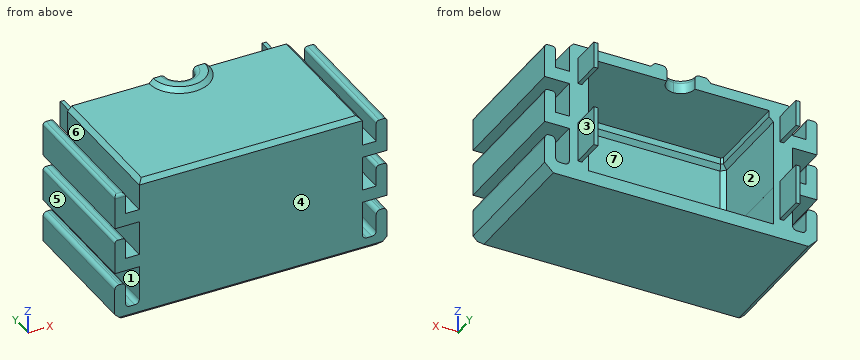
```python
from build123d import *

# Parameters (mm, degrees)
ESQUISSE1_W              = 51.86
ESQUISSE1_H              = 63
BOSS_EXTRU_1_DEPTH       = 20
ENL_V_MAT_EXTRU_1_DEPTH  = 18
ESQUISSE3_W              = 8.7
ESQUISSE3_H              = 3
BOSS_EXTRU_2_DEPTH       = 7
ESQUISSE4_W              = 43
ESQUISSE4_H              = 43
BOSS_EXTRU_3_DEPTH       = 1
CHANFREIN1_SIZE          = 1
ESQUISSE6_R              = 7
BOSS_EXTRU_4_DEPTH       = 5
ENL_V_MAT_EXTRU_2_DEPTH  = 10
BOSS_EXTRU_5_DEPTH       = 63
ESQUISSE9_W              = 2.5
ESQUISSE9_H              = 1
ENL_V_MAT_EXTRU_3_DEPTH  = 63
CHANFREIN3_SIZE          = 1
CONG_1_R                 = 1
CONG_2_R                 = 1
CONG_5_R                 = 0.7
ENL_V_MAT_EXTRU_11_DEPTH = 1.5
ESQUISSE24_W             = 38.565319184
ESQUISSE24_H             = 34.907409987
ENL_V_MAT_EXTRU_16_DEPTH = 74
BOSS_EXTRU_11_REACH      = 71.206
ESQUISSE26_W             = 43.000682915
ESQUISSE26_H             = 8.323167201
ENL_V_MAT_EXTRU_17_DEPTH = 74
ESQUISSE27_W             = 43.00063515
ESQUISSE27_H             = 9
BOSS_EXTRU_12_DEPTH      = 10
BOSS_EXTRU_13_DEPTH      = 1
CHANFREIN4_SIZE          = 1
CHANFREIN5_SIZE          = 1
ESQUISSE29_W             = 0.940494366
ESQUISSE29_H             = 6.11321338
ESQUISSE29_H_2           = 9.278042655
BOSS_EXTRU_14_DEPTH      = 7


with BuildPart() as part:
    # Esquisse1 → Boss.-Extru.1 (new body)
    with BuildSketch(Plane.XY):
        with Locations((25.93, 31.5)):
            Rectangle(ESQUISSE1_W, ESQUISSE1_H)
    extrude(amount=BOSS_EXTRU_1_DEPTH)

    # Esquisse2 → Enlèv. mat.-Extru.1 (cut)
    with BuildSketch(Plane(origin=(0, 0, 0), x_dir=(-1, 0, 0), z_dir=(0, 0, -1))):
        Polygon((-8.231746032, 10), (-43.628253968, 53), (-47.43, 53), (-47.43, 10), align=None)
        Polygon((-4.43, 53), (-43.628253968, 53), (-8.231746032, 10), (-4.43, 10), align=None)
    extrude(amount=-ENL_V_MAT_EXTRU_1_DEPTH, mode=Mode.SUBTRACT)

    # Esquisse3 → Boss.-Extru.2 (add)
    with BuildSketch(Plane(origin=(0, 0, 0), x_dir=(-1, 0, 0), z_dir=(0, 0, -1))):
        with Locations((-8.88, 57.4)):
            Rectangle(ESQUISSE3_W, ESQUISSE3_H)
        with Locations((-42.98, 57.4)):
            Rectangle(ESQUISSE3_W, ESQUISSE3_H)
        with Locations((-42.98, 5.6)):
            Rectangle(ESQUISSE3_W, ESQUISSE3_H)
        with Locations((-8.88, 5.6)):
            Rectangle(ESQUISSE3_W, ESQUISSE3_H)
    extrude(amount=BOSS_EXTRU_2_DEPTH)

    # Esquisse4 → Boss.-Extru.3 (add)
    with BuildSketch(Plane(origin=(0, 0, 18), x_dir=(-1, 0, 0), z_dir=(0, 0, -1))):
        with Locations((-25.93, 31.5)):
            Rectangle(ESQUISSE4_W, ESQUISSE4_H)
    extrude(amount=BOSS_EXTRU_3_DEPTH)

    # Chanfrein1
    chanfrein1_edges = [part.edges().sort_by_distance(p)[0] for p in [
        (47.43, 10, 8.5),
        (47.43, 53, 8.5),
        (4.43, 10, 8.5),
        (4.43, 53, 8.5),
    ]]
    chamfer(chanfrein1_edges, length=CHANFREIN1_SIZE)

    # Esquisse6 → Boss.-Extru.4 (add)
    with BuildSketch(Plane(origin=(0, 0, 17), x_dir=(-1, 0, 0), z_dir=(0, 0, -1))):
        with Locations((-25.93, 31.5)):
            Circle(ESQUISSE6_R)
    extrude(amount=-BOSS_EXTRU_4_DEPTH)

    # Esquisse7 → Enlèv. mat.-Extru.2 (cut)
    with BuildSketch(Plane(origin=(0, 0, 17), x_dir=(-1, 0, 0), z_dir=(0, 0, -1))):
        with BuildLine():
            ThreePointArc((-22.68, 31.5), (-23.631902961, 33.798097039), (-25.93, 34.75))
            Line((-25.93, 34.75), (-25.93, 28.25))
            ThreePointArc((-25.93, 28.25), (-23.631902961, 29.201902961), (-22.68, 31.5))
        make_face()
        with BuildLine():
            Line((-25.93, 28.25), (-25.93, 34.75))
            ThreePointArc((-25.93, 34.75), (-29.18, 31.5), (-25.93, 28.25))
        make_face()
    extrude(amount=-ENL_V_MAT_EXTRU_2_DEPTH, mode=Mode.SUBTRACT)

    # Esquisse8 → Boss.-Extru.5 (add)
    with BuildSketch(Plane(origin=(0, 63, 0), x_dir=(1, 0, 0), z_dir=(0, 1, 0))):
        Polygon((55.06, -3), (55.06, -9), (57.56, -9), (57.56, 0), (51.86, 0), (51.86, -3), align=None)
        Polygon((57.56, -11), (51.86, -11), (51.86, -14), (55.06, -14), (55.06, -20), (57.56, -20), align=None)
        Polygon((0, -3), (0, 0), (-5.7, 0), (-5.7, -9), (-3.2, -9), (-3.2, -3), align=None)
        Polygon((0, -14), (0, -11), (-5.7, -11), (-5.7, -20), (-3.2, -20), (-3.2, -14), align=None)
    extrude(amount=-BOSS_EXTRU_5_DEPTH)

    # Esquisse9 → Enlèv. mat.-Extru.3 (cut)
    with BuildSketch(Plane.XZ):
        with Locations((-4.45, 8.5)):
            Rectangle(ESQUISSE9_W, ESQUISSE9_H)
        with Locations((-4.45, 19.5)):
            Rectangle(ESQUISSE9_W, ESQUISSE9_H)
        with Locations((56.31, 8.5)):
            Rectangle(ESQUISSE9_W, ESQUISSE9_H)
        with Locations((56.31, 19.5)):
            Rectangle(ESQUISSE9_W, ESQUISSE9_H)
    extrude(amount=-ENL_V_MAT_EXTRU_3_DEPTH, mode=Mode.SUBTRACT)

    # Chanfrein3
    chanfrein3_edges = [part.edges().sort_by_distance(p)[0] for p in [
        (46.93, 52.5, 17),
        (4.93, 52.5, 17),
        (46.93, 10.5, 17),
        (4.93, 10.5, 17),
        (25.93, 34.75, 17),
        (4.43, 31.5, 17),
        (25.93, 10, 17),
        (47.43, 31.5, 17),
        (25.93, 53, 17),
    ]]
    chamfer(chanfrein3_edges, length=CHANFREIN3_SIZE)

    # Congé1
    cong_1_edges = [part.edges().sort_by_distance(p)[0] for p in [
        (4.53, 57.4, -7),
        (8.88, 55.9, -7),
        (8.88, 58.9, -7),
        (13.23, 57.4, -7),
        (38.63, 57.4, -7),
        (42.98, 58.9, -7),
        (47.33, 57.4, -7),
        (42.98, 55.9, -7),
        (47.33, 5.6, -7),
        (42.98, 7.1, -7),
        (42.98, 4.1, -7),
        (38.63, 5.6, -7),
        (13.23, 5.6, -7),
        (8.88, 4.1, -7),
        (4.53, 5.6, -7),
        (8.88, 7.1, -7),
    ]]
    fillet(cong_1_edges, radius=CONG_1_R)

    # Congé2
    cong_2_edges = [part.edges().sort_by_distance(p)[0] for p in [
        (25.93, 34.75, 22),
    ]]
    fillet(cong_2_edges, radius=CONG_2_R)

    # Congé5
    cong_5_edges = [part.edges().sort_by_distance(p)[0] for p in [
        (-3.2, 31.5, 19),
        (-5.7, 31.5, 19),
        (-3.2, 31.5, 8),
        (-5.7, 31.5, 8),
        (55.06, 31.5, 8),
        (57.56, 31.5, 8),
        (55.06, 31.5, 19),
        (57.56, 31.5, 19),
        (-4.45, 0, 19),
        (-4.45, 63, 19),
    ]]
    fillet(cong_5_edges, radius=CONG_5_R)

    # Esquisse19 → Enlèv. mat.-Extru.11 (cut)
    with BuildSketch(Plane(origin=(0, 0, 17), x_dir=(-1, 0, 0), z_dir=(0, 0, -1))):
        Polygon((-46.43, 11.414213562), (-46.015786438, 11), (-5.844213562, 11), (-5.43, 11.414213562), (-5.43, 51.585786438), (-5.844213562, 52), (-46.015786438, 52), (-46.43, 51.585786438), align=None)
    extrude(amount=-ENL_V_MAT_EXTRU_11_DEPTH, mode=Mode.SUBTRACT)

    # Esquisse24 → Enlèv. mat.-Extru.16 (cut)
    with BuildSketch(Plane(origin=(57.56, 0, 0), x_dir=(0, 0, -1), z_dir=(1, 0, 0))):
        with Locations((-11.348740569, 48.953704994)):
            Rectangle(ESQUISSE24_W, ESQUISSE24_H)
    extrude(amount=-ENL_V_MAT_EXTRU_16_DEPTH, mode=Mode.SUBTRACT)

    # Boss.-Extru.11: up to this face of the body (flat: up to its plane)
    boss_extru_11_end = Plane(part.part.faces().sort_by_distance((25.97056106, 0, 9.851467598))[0])
    # Esquisse25 → Boss.-Extru.11 (add, up to the picked face)
    with BuildSketch(Plane(origin=(0, 31.5, 0), x_dir=(1, 0, 0), z_dir=(0, 1, 0)), mode=Mode.PRIVATE) as boss_extru_11_sk1:
        with BuildLine():
            Line((47.42936485, 9), (47.43, 0))
            Line((47.43, 0), (51.86, 0))
            Line((51.86, 0), (51.86, 8))
            ThreePointArc((51.86, 8), (52.152893219, 8.707106781), (52.86, 9))
            Line((52.86, 9), (54.06, 9))
            ThreePointArc((54.06, 9), (54.767106781, 8.707106781), (55.06, 8))
            Line((55.06, 8), (55.06, 4))
            ThreePointArc((55.06, 4), (55.352893219, 3.292893219), (56.06, 3))
            Line((56.06, 3), (56.56, 3))
            ThreePointArc((56.56, 3), (57.267106781, 3.292893219), (57.56, 4))
            Line((57.56, 4), (57.56, 10))
            Line((57.56, 10), (55.56, 12))
            Line((55.56, 12), (25.92936485, 12))
            Line((25.92936485, 12), (25.92936485, 9))
            Line((25.92936485, 9), (47.42936485, 9))
        make_face()
    boss_extru_11_tool1 = split(extrude(boss_extru_11_sk1.sketch, amount=-BOSS_EXTRU_11_REACH, mode=Mode.PRIVATE), bisect_by=boss_extru_11_end, keep=Keep.BOTH, mode=Mode.PRIVATE)
    # Esquisse25 → Boss.-Extru.11 (add, up to the picked face)
    with BuildSketch(Plane(origin=(0, 31.5, 0), x_dir=(1, 0, 0), z_dir=(0, 1, 0)), mode=Mode.PRIVATE) as boss_extru_11_sk2:
        with BuildLine():
            Line((4.42936485, 9), (25.92936485, 9))
            Line((25.92936485, 9), (25.92936485, 12))
            Line((25.92936485, 12), (-3.7012703, 12))
            Line((-3.7012703, 12), (-5.7012703, 10))
            Line((-5.7012703, 10), (-5.7012703, 4))
            ThreePointArc((-5.7012703, 4), (-5.408377081, 3.292893219), (-4.7012703, 3))
            Line((-4.7012703, 3), (-4.2012703, 3))
            ThreePointArc((-4.2012703, 3), (-3.494163519, 3.292893219), (-3.2012703, 4))
            Line((-3.2012703, 4), (-3.2012703, 8))
            ThreePointArc((-3.2012703, 8), (-2.908377081, 8.707106781), (-2.2012703, 9))
            Line((-2.2012703, 9), (-1.0012703, 9))
            ThreePointArc((-1.0012703, 9), (-0.294163519, 8.707106781), (-0.0012703, 8))
            Line((-0.0012703, 8), (-0.0012703, 0))
            Line((-0.0012703, 0), (4.4287297, 0))
            Line((4.4287297, 0), (4.42936485, 9))
        make_face()
    boss_extru_11_tool2 = split(extrude(boss_extru_11_sk2.sketch, amount=-BOSS_EXTRU_11_REACH, mode=Mode.PRIVATE), bisect_by=boss_extru_11_end, keep=Keep.BOTH, mode=Mode.PRIVATE)
    add(boss_extru_11_tool1.solids().sort_by(Axis((36.679365, 31.5, -9.338304), (0, -1, 0)))[0])
    add(boss_extru_11_tool2.solids().sort_by(Axis((15.179365, 31.5, -9.338304), (0, -1, 0)))[0])

    # Esquisse26 → Enlèv. mat.-Extru.17 (cut)
    with BuildSketch(Plane.XZ.offset(-4.1)):
        with Locations((25.929658543, -4.161583601)):
            Rectangle(ESQUISSE26_W, ESQUISSE26_H)
    extrude(amount=-ENL_V_MAT_EXTRU_17_DEPTH, mode=Mode.SUBTRACT)

    # Esquisse27 → Boss.-Extru.12 (add)
    with BuildSketch(Plane.XZ):
        with Locations((25.929682425, -4.5)):
            Rectangle(ESQUISSE27_W, ESQUISSE27_H)
    extrude(amount=-BOSS_EXTRU_12_DEPTH)

    # Esquisse28 → Boss.-Extru.13 (add)
    with BuildSketch(Plane.XY.offset(20)):
        with BuildLine():
            Line((51.86, 0), (51.86, 31.5))
            Line((51.86, 31.5), (32.93, 31.5))
            ThreePointArc((32.93, 31.5), (25.93, 24.5), (18.93, 31.5))
            Line((18.93, 31.5), (0, 31.5))
            Line((0, 31.5), (0, 0))
            Line((0, 0), (51.86, 0))
        make_face()
    extrude(amount=BOSS_EXTRU_13_DEPTH)

    # Chanfrein4
    chanfrein4_edges = [part.edges().sort_by_distance(p)[0] for p in [
        (25.93, 24.5, 22),
    ]]
    chamfer(chanfrein4_edges, length=CHANFREIN4_SIZE - 0.0001)  # a hair under: the kernel refuses the full size

    # Chanfrein5
    chanfrein5_edges = [part.edges().sort_by_distance(p)[0] for p in [
        (25.92936485, 0, -12),
        (25.93, 0, 21),
        (51.86, 15.75, 21),
        (0, 15.75, 21),
    ]]
    chamfer(chanfrein5_edges, length=CHANFREIN5_SIZE)

    # Esquisse29 → Boss.-Extru.14 (add)
    with BuildSketch(Plane(origin=(0, 31.5, 0), x_dir=(1, 0, 0), z_dir=(0, 1, 0))):
        with Locations((2.465352228, -14.677342748)):
            Rectangle(ESQUISSE29_W, ESQUISSE29_H)
        with Locations((2.465352228, 2.720621555)):
            Rectangle(ESQUISSE29_W, ESQUISSE29_H_2)
        with Locations((49.394647772, 2.720621555)):
            Rectangle(ESQUISSE29_W, ESQUISSE29_H_2)
        with Locations((49.394647772, -14.677342748)):
            Rectangle(ESQUISSE29_W, ESQUISSE29_H)
    extrude(amount=BOSS_EXTRU_14_DEPTH)


solid = part.part
```
Build history of the part. All positions in model axes, mm. Face numbers are marked on the shaded views. A direction names the side the tool comes from. Round coordinates to 2 decimals unless told otherwise and drop trailing zeros. Write each loop counter-clockwise with the first axis right and the second up, starting at its lowest first coordinate (ties: lowest second). Pieces come first, ordered by that corner, then holes.
1) Pin check, flat tips, straight feed: pin 1 (2 mm diameter, centred on y = 34, z = -2, fed in from +X); pin 2 (0.8 mm diameter, centred on x = 2.5, y = 34, fed in from -Z); pin 3 (0.5 mm diameter, centred on x = 49.5, y = 35, fed in from +Z). Stop position of each tip, or through.
2) Mould opens along X. For the marked faces 4, 5, 6 and 7 say: +X half, -X half, draft (parallel to the pull), parting line (faces both ways), or undercut.
3) Band-saw the part on A-A, the plane z = 13. List the corners of the cut face in (x, y).
4) 3-axis set-ups, long thin cutter, end or side, ignore diameter. For the marked faces 1, 2 and 3: which of +Z, -Z, +X, -X, +Y, -Y reach the whole face in a straight line?
5) Drill centre lines: probe 1 along X at (y, z) = (24, 7); probe 2 along X at (y, z) = (8, 5); probe 3 along Z at (x, y) = (-1.5, 23.5). Where is each one in solid material? Low to high.
6) Band-saw the part on B-B, the plane z = -2. List the corners of the cut face in (x, y).
Ans:
1. pin 1: stops at x = 49.86
1. pin 2: stops at z = -7.36
1. pin 3: stops at z = 17.73
2. face 4: draft
2. face 5: -X half
2. face 6: undercut
2. face 7: undercut
3. outline: (-5.7, 0) - (57.56, 0) - (57.56, 31.5) - (49.86, 31.5) - (49.86, 38.5) - (48.92, 38.5) - (48.92, 31.5) - (47.43, 31.5) - (47.43, 11) - (46.43, 10) - (5.43, 10) - (4.43, 11) - (4.43, 31.5) - (2.94, 31.5) - (2.94, 38.5) - (2, 38.5) - (2, 31.5) - (-5.7, 31.5) - close
4. face 1: +Y, -Y
4. face 2: +Y
4. face 3: +Z, -Z, +X, +Y
5. probe 1: x = -5.7 to -3.2, 0 to 4.43, 47.43 to 51.86, 55.06 to 57.56
5. probe 2: x = -5.7 to -3.2, 0 to 51.86, 55.06 to 57.56
5. probe 3: z = -12 to -9, 0 to 3, 11 to 14
6. outline: (0, 0) - (4.43, 0) - (4.43, 31.5) - (2.94, 31.5) - (2.94, 38.5) - (2, 38.5) - (2, 31.5) - (0, 31.5) - close; (4.43, 0) - (51.86, 0) - (51.86, 31.5) - (49.86, 31.5) - (49.86, 38.5) - (48.92, 38.5) - (48.92, 31.5) - (47.43, 31.5) - (47.43, 10) - (4.43, 10) - close
